Here's how the part is built. I have some questions about the finished solid (model axes, mm). Give positions to 0.01 mm unless a question says otherwise; leave off trailing zeros. Write each loop counter-clockwise with the first axis right and the second up, starting at its lowest first coordinate (ties: lowest second). Pieces come first, ordered by that corner, then holes. Notation, with made-up numbers: (-24, -9.75) - (2, -9.75) arc R21 ccw to (2, 4.25) - close; hole circle Ø9 at (18, 56). An arc over 180 degrees is marked (long way). Use a Markdown table: item, result.
Autodesk Inventor part; units mm, degrees
ref_plane "YZ Plane" through (0, 0, 0) normal (1, 0, 0) x (0, 1, 0)
ref_plane "XZ Plane" through (0, 0, 0) normal (0, 1, 0) x (-1, 0, 0)
ref_plane "XY Plane" through (0, 0, 0) normal (0, 0, 1) x (1, 0, 0)
sketch "スケッチ2" plane through (0, 0, 0) normal (0, 1, 0) x (-1, 0, 0)
  line L0 (-32.5, -11.25) -> (32.5, -11.25)
  line L1 (32.5, -11.25) -> (32.5, 11.25)
  line L2 (32.5, 11.25) -> (-32.5, 11.25)
  line L3 (-32.5, 11.25) -> (-32.5, -11.25)
  line L4 (-32.5, -11.25) -> (32.5, 11.25) construction
  line L5 (32.5, -11.25) -> (-32.5, 11.25) construction
  line L6 (-30, -8.75) -> (30, -8.75)
  line L7 (30, -8.75) -> (30, 8.75)
  line L8 (30, 8.75) -> (-30, 8.75)
  line L9 (-30, 8.75) -> (-30, -8.75)
  line L10 (-30, -8.75) -> (30, 8.75) construction
  line L11 (30, -8.75) -> (-30, 8.75) construction
  circle A0 centre (30, 8.75) radius 2.5
  circle A1 centre (30, -8.75) radius 2.5
  circle A2 centre (-30, 8.75) radius 2.5
  circle A3 centre (-30, -8.75) radius 2.5
  line L12 (-115, -18.25) -> (115, -18.25)
  line L13 (115, -18.25) -> (115, 18.25)
  line L14 (115, 18.25) -> (-115, 18.25)
  line L15 (-115, 18.25) -> (-115, -18.25)
  line L16 (-115, -18.25) -> (115, 18.25) construction
  line L17 (115, -18.25) -> (-115, 18.25) construction
  line L18 (-95, -18.25) -> (95, -18.25)
  line L19 (95, -18.25) -> (95, 18.25)
  line L20 (95, 18.25) -> (-95, 18.25)
  line L21 (-95, 18.25) -> (-95, -18.25)
  line L22 (-95, -18.25) -> (95, 18.25) construction
  line L23 (95, -18.25) -> (-95, 18.25) construction
  point P0 (0, 0)
  dimension "d10" = 65
  dimension "d11" = 22.5
  dimension "d12" = 60
  dimension "d13" = 17.5
  dimension "d14" = 230
  dimension "d15" = 36.5
  dimension "d16" = 190
sketch "スケッチ4" plane through (0, 0, 0) normal (1, 0, 0) x (0, 1, 0)
  point P0 (0, 0)
sketch "スケッチ5" plane through (0, 0, 0) normal (1, 0, 0) x (0, 1, 0)
  circle A0 centre (0, 0) radius 18.25
  line L0 (0, 0) -> (0, 6)
  line L1 (0, 6) -> (0, -6)
  circle A1 centre (0, 6) radius 3
  circle A2 centre (0, -6) radius 9
  circle A3 centre (0, 6) radius 9
  circle A4 centre (0, -6) radius 3
  line L2 (0, 6) -> (5.2915, 0)
  circle A5 centre (5.2915, 0) radius 5
  circle A6 centre (5.2915, 0) radius 4.5
  circle A7 centre (5.2915, 0) radius 5.5
  line L3 (0, 0) -> (0, 11.25)
  line L4 (0, 11.25) -> (0, -11.25)
  line L5 (5.2915, 5.5) -> (5.2915, -5.5)
  line L6 (0, 11.25) -> (-1.2, 11.25)
  line L7 (-1.2, 11.25) -> (-1.2, -11.25)
  line L8 (-1.2, -11.25) -> (0, -11.25)
  line L9 (-1.2, 11.25) -> (-9.2, 11.25)
  line L10 (-1.2, -11.25) -> (-9.2, -11.25)
  line L11 (-9.2, -11.25) -> (-9.2, 11.25)
  line L12 (-9.2, 11.25) -> (-10.4, 11.25)
  line L13 (-10.4, 11.25) -> (-10.4, -11.25)
  line L14 (-10.4, -11.25) -> (-9.2, -11.25)
  circle A8 centre (0, 0) radius 16
  line L15 (0, 11.25) -> (1.5, 11.25)
  line L16 (1.5, 11.25) -> (1.5, -11.25)
  line L17 (1.5, -11.25) -> (0, -11.25)
  line L18 (5.2915, 5.5) -> (1.5, 5.5)
  line L19 (5.2915, -5.5) -> (1.5, -5.5)
  circle A9 centre (5.2915, 0) radius 6.6802
  point P0 (0, 1.5)
  point P1 (0, -1.5)
  point P2 (1.5, -3.9843)
  point P3 (1.5, 3.9843)
  dimension "d28" = 36.5
  dimension "d29" = 6
  dimension "d30" = 12
  dimension "d31" = 6
  dimension "d32" = 18
  dimension "d33" = 8
  dimension "d34" = 9
  dimension "d35" = 11
  dimension "d36" = 11.25
  dimension "d37" = 22.5
  dimension "d39" = 1.2
  dimension "d40" = 8
  dimension "d41" = 1.2
  dimension "d42" = 32
  dimension "d43" = 1.5
ref_plane "作業平面1" through (16.5, 5.2915, 0) normal (1, 0, 0) x (0, 0, 1)
sketch "スケッチ6" plane through (16.5, 5.2915, 0) normal (1, 0, 0) x (0, 0, 1)
  line L0 (0, 5.2915) -> (6, 5.2915)
  line L1 (-11.25, 5.2915) -> (11.25, 5.2915)
  line L2 (6, 5.2915) -> (-6, 5.2915)
  circle A0 centre (6, 5.2915) radius 1.25
  circle A1 centre (-6, 5.2915) radius 1.25
  circle A2 centre (0, 5.2915) radius 16
  circle A3 centre (0, 0) radius 5
  line L3 (0, 0) -> (0, 3)
  line L4 (0, 3) -> (0, -5.5)
  arc A4 (-5.5, 0) -> (5.5, 0) centre (0, 0) ccw
  line L5 (0, 3) -> (1, 3)
  line L6 (1, 3) -> (-1, 3)
  line L7 (-1, 3) -> (-1, -5.4083)
  line L8 (1, 3) -> (1, -5.4083)
  circle A5 centre (6, 5.2915) radius 9
  circle A6 centre (-6, 5.2915) radius 9
  line L9 (0, 5.2915) -> (0, -2.7085)
  circle A7 centre (0, -2.7085) radius 8
  circle A8 centre (6, 5.2915) radius 10
  circle A9 centre (-6, 5.2915) radius 10
  line L10 (0, 5.2915) -> (0, -5.7085)
  line L11 (0, -5.7085) -> (-11.619, -5.7085)
  line L12 (0, -5.7085) -> (11.619, -5.7085)
  line L13 (0, -5.7085) -> (9.5, -5.7085)
  line L14 (9.5, -5.7085) -> (-9.5, -5.7085)
  circle A10 centre (0, 5.2915) radius 18
  line L15 (1, -5.4083) -> (1, -8.2085)
  line L16 (-1, -5.4083) -> (-1, -8.2085)
  line L17 (0, 5.2915) -> (0, 6.4915)
  line L18 (0, 6.4915) -> (0, 14.4915)
  line L19 (0, 14.4915) -> (0, 15.6915)
  line L20 (0, 15.6915) -> (-11.25, 15.6915)
  line L21 (-11.25, 15.6915) -> (11.25, 15.6915)
  line L22 (11.25, 15.6915) -> (11.25, 14.4915)
  line L23 (11.25, 14.4915) -> (0, 14.4915)
  line L24 (-11.25, 14.4915) -> (-11.25, 15.6915)
  line L25 (0, 14.4915) -> (-11.25, 14.4915)
  line L26 (0, 15.6915) -> (8.75, 15.6915)
  line L27 (8.75, 15.6915) -> (-8.75, 15.6915)
  line L28 (11.25, 15.6915) -> (11.25, 17.1915)
  line L29 (11.25, 17.1915) -> (-11.25, 17.1915)
  line L30 (-11.25, 17.1915) -> (-11.25, 15.6915)
  line L31 (6, 17.1915) -> (6, 18.6915)
  line L32 (-6, 17.1915) -> (-6, 18.6915)
  circle A11 centre (6, 18.6915) radius 2.5
  circle A12 centre (-6, 18.6915) radius 2.5
  line L33 (6, 21.1915) -> (-6, 21.1915)
  line L34 (9.5, -5.7085) -> (12, -5.7085)
  line L35 (-9.5, -5.7085) -> (-12, -5.7085)
  line L36 (6, 18.6915) -> (8.5, 18.6915)
  line L37 (-6, 18.6915) -> (-8.5, 18.6915)
  circle A13 centre (0, 0) radius 4.5
  circle A14 centre (-6, 5.2915) radius 1.5
  circle A15 centre (6, 5.2915) radius 1.5
  circle A16 centre (6, 18.6915) radius 1.65
  circle A17 centre (-6, 18.6915) radius 1.65
  line L38 (9.5, -5.7085) -> (9.5, -6.2085)
  line L39 (9.5, -6.2085) -> (-9.5, -6.2085)
  line L40 (-9.5, -6.2085) -> (-9.5, -5.7085)
  circle A18 centre (-9.5, -6.2085) radius 1.65
  circle A19 centre (9.5, -6.2085) radius 1.65
  circle A20 centre (9.5, -6.2085) radius 2.5
  circle A21 centre (-9.5, -6.2085) radius 2.5
  line L41 (-12, -6.2085) -> (-8.5, 18.6915)
  line L42 (12, -6.2085) -> (8.5, 18.6915)
  line L43 (9.5, -8.7085) -> (-9.5, -8.7085)
  line L44 (1, -8.7085) -> (1, -8.0358)
  line L45 (-1, -8.7085) -> (-1, -8.2085)
  point P0 (1, -4.3875)
  point P1 (-1, -4.3875)
  point P2 (-4.4567, 20.6583)
  point P3 (-8.495, 18.8501)
  point P4 (4.4567, 20.6583)
  point P5 (8.495, 18.8501)
  point P6 (1.7861, 21.1915)
  point P7 (-1.7861, 21.1915)
  point P8 (11.9031, -5.5193)
  point P9 (11.8759, -5.4306)
  point P10 (11.8887, -5.4164)
  dimension "d54" = 6
  dimension "d55" = 12
  dimension "d56" = 2.5
  dimension "d57" = 2.5
  dimension "d58" = 32
  dimension "d59" = 10
  dimension "d60" = 3
  dimension "d61" = 1
  dimension "d62" = 2
  dimension "d65" = 18
  dimension "d66" = 18
  dimension "d67" = 8
  dimension "d68" = 11
  dimension "d69" = 9.5
  dimension "d70" = 19
  dimension "d73" = 36
  dimension "d76" = 1.2
  dimension "d77" = 8
  dimension "d78" = 1.2
  dimension "d79" = 8.75
  dimension "d80" = 17.5
  dimension "d81" = 1.5
  dimension "d82" = 1.5
  dimension "d83" = 5
  dimension "d84" = 5
  dimension "d97" = 3
  dimension "d98" = 3
  dimension "d109" = 3.3
  dimension "d110" = 3.3
  dimension "d111" = 0.5
  dimension "d112" = 3.3
  dimension "d113" = 3.3
  dimension "d114" = 5
  dimension "d115" = 5
extrude "押し出し11" add sketch "スケッチ6" against normal blind 4 contours L17 L18 A6 L0 | A7 A5 L1 | A7 A6 A3 L9 | L0 A6 A7 | L9 A3 A5 A7 | L1 A5 L18 L17 | A6 A5 A9 L0 | L0 A9 A7 A6 | A5 A7 A8 L1 | L1 A8 A6 A5 | L9 A13 A5 A3 | A3 A6 A13 L9 | A7 A9 A3 A6 | A5 A3 A8 A7 | A9 A5 L42 L1 A15 L0 | L0 A15 L1 L42 A5 A7 A9 | L18 A9 A5 | A6 A8 L18 | A8 A7 A6 L41 L1 A14 | L1 A14 L41 A6 A8 | A3 A9 A13 A6 | A5 A13 A8 A3 | A13 A6 L8 L5 L9 | L9 L6 L7 A5 A13 | A7 A5 A3 A9 | A8 A3 A6 A7 | A15 L1 A0 L0 | L0 A0 L1 A15 | A9 A8 L23 L42 A5 | A6 L41 L25 A9 A8 | L18 L23 A8 | A9 L25 L18 | A14 L1 A1 | L1 A1 A14 | A3 A5 A13 A9 | A13 A9 L8 A6 | A8 A13 A6 A3 | A5 L7 A8 A13 | L5 L8 A6 L4 L3 | L3 L4 A5 L7 L6 | A7 A21 A9 L41 A6 | A6 A4 A9 A21 A7 | L23 L19 L21 L42 A8 | A8 L42 L23 | L25 L41 A9 | A9 L41 L20 L19 L25 | A13 A5 L8 A9 | L8 A9 A5 A6 | A6 A13 A9 A3 | A3 A9 A4 A6 | A8 L7 A6 A13 | A5 A6 A8 L7 | A7 A20 A8 A4 A5 | A5 L42 A8 A20 A7 | A21 A9 A7 | A7 A9 A21 | L20 L41 L29 A12 A11 L42 L21 | A5 A4 A8 A3 | A3 A8 A13 A5 | L8 A5 A9 | A5 A9 L4 | L4 A8 A6 | A9 A13 L7 A3 | A3 L7 A4 A9 | A6 L7 A9 A13 | A8 A6 L7 | A20 A8 A7 | A7 A8 A20 | A9 A21 A2 L41 | A4 L16 L11 A21 A9 | A9 A21 L11 A7 | A7 L11 A18 A2 A21 A9 | A8 A4 L8 A3 | A3 L8 A13 A8 | A13 A8 L8 A5 | L8 A8 A9 A5 | A8 L8 A13 L4 | A9 L7 A6 A8 | L4 A13 L7 A9 | L7 A13 L4 A3 | A3 L4 A4 L7 | A9 L7 A13 | A8 A20 L12 L15 A4 | L42 A2 A20 A8 | A8 A20 A2 L12 A19 A7 | A7 L12 A20 A8 | A2 A21 L41 | A4 L10 L11 L16 | L11 A21 L39 A7 | A7 L39 A18 L11 | L11 L16 L39 A21 | A2 L35 L41 A21 | L29 A11 L42 | L41 A12 L29 | L8 A4 L4 A3 | A3 L4 A13 L8 | A13 L8 A8 | L15 L12 L10 A4 | L12 A19 L39 A7 | A7 L39 A20 L12 | A20 L42 L34 A2 | A20 L39 L15 L12 | L11 L12 L15 L39 L16 | L39 A21 A7 | A7 A21 A2 A18 L39 | L39 L16 L45 L43 A7 A21 | L11 A18 A2 | A2 A18 A21 L41 L35 | A11 L29 A16 | L29 A16 L36 A11 | L36 A16 A2 A11 | A12 L37 A17 L29 | L29 A17 A12 | A12 A2 A17 L37 | L39 A19 A2 A20 A7 | A7 A20 L39 | L34 L42 A20 A2 A19 | A2 A19 L12 | A20 A7 L43 L44 L15 L39 | L39 L15 L44 L43 L45 L16 | A7 L43 A2 A21 | A2 A16 A11 | A11 A2 A16 L29 | L29 A12 A2 L33 A11 | L29 A17 A2 A12 | A12 A2 A17 | A20 A2 L43 A7 | A2 L43 A21 | A11 A2 L33 | L33 A2 A12 | A20 L43 A2 picked at (5.1751, 14.7127) picked at (-5.1751, 14.7127)
hole "穴2" at (16.5, 0, 0) direction (-1, 0, 0) diameter 3.3 end through all
properties part number "ikafly1b"
Item 1: If we section it at A-A, the plane x = 13.45: Count the separate pieces of the cut face and the enclosed holes in it, plus the area to 3 significant figures.
Values:
| item | result |
|---|---|
| separate pieces | 1 |
| enclosed holes | 7 |
| area | 555 mm2 |
Item 2: I need wall thicknesses on line 1 along Y through (x, z) = (13.4, -6); line 2 along Z through (x, y) = (14.6, -13.4); line 3 along Z through (x, y) = (13.3, 11.5). Which ranges of each line are inside material? Lowest first, please. Write a range as [from, to].
Values:
| item | result |
|---|---|
| line 1 | y = [-15.9, -15.05], [-11.75, -1.25], [1.25, 14] |
| line 2 | z = [-8.5, -7.65], [-4.35, 4.35], [7.65, 8.5] |
| line 3 | z = [-12, -11.15], [-7.85, 7.85], [11.15, 12] |
Item 3: Will this pin go through, and if not, where does the flat tip stop? pin 1 Ø1 at (x, y) = (13.5, -6.5) entering from -Z.
Values:
| item | result |
|---|---|
| pin 1 | stops at z = -9.54 |
Item 4: If we section it at D-D, the plane z = -1.25: Write out the boundary of the cut face in (x, y), plus the area to 3 significant figures.
Values:
| item | result |
|---|---|
| outline | (12.5, -15.9) - (16.5, -15.9) - (16.5, -1.08) - (12.5, -1.08) - close; (12.5, 1.08) - (16.5, 1.08) - (16.5, 14) - (12.5, 14) - close |
| area | 111 mm2 |
Item 5: Thinking about a two-plate mould opening in Y: for faces 1 (the flat face through (14.528, -0.776, -10.274)), 2 (the cylindrical face through (14.528, 13.248, -11.287)), 3 (the cylindrical face through (14.5, 13.1, 9.1)), which applies, +Y half, -Y half, draft (parallel to the pull), parting line (faces both ways), or undercut?
Values:
| item | result |
|---|---|
| face 1 | -Y half |
| face 2 | +Y half |
| face 3 | undercut |
Item 6: If we section it at B-B, the plane z = 9: Write out the boundary of the cut face in (x, y), plus the area to 3 significant figures.
Values:
| item | result |
|---|---|
| outline | (12.5, -9.84) - (16.5, -9.84) - (16.5, 9.93) - (12.5, 9.93) - close; (12.5, 13.07) - (16.5, 13.07) - (16.5, 14) - (12.5, 14) - close |
| area | 82.8 mm2 |
Item 7: If we section it at C-C, the plane y = 0.5: Write out the boundary of the cut face in (x, z).
Values:
| item | result |
|---|---|
| outline | (12.5, -10.45) - (16.5, -10.45) - (16.5, -7.15) - (12.5, -7.15) - close; (12.5, -4.85) - (16.5, -4.85) - (16.5, -1.57) - (12.5, -1.57) - close; (12.5, 1.57) - (16.5, 1.57) - (16.5, 4.85) - (12.5, 4.85) - close; (12.5, 7.15) - (16.5, 7.15) - (16.5, 10.45) - (12.5, 10.45) - close |
